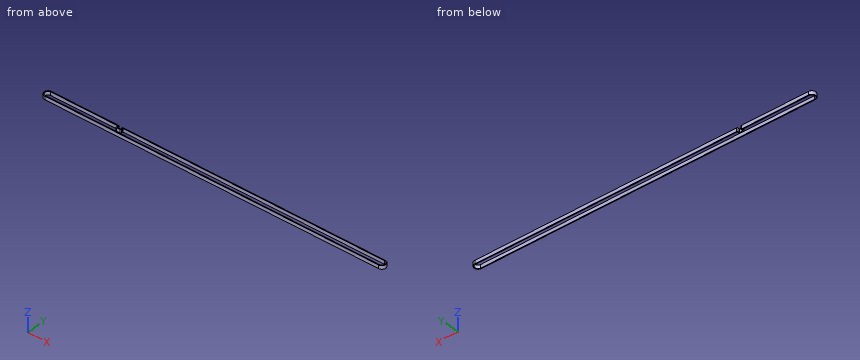
```python
from build123d import *

# Parameters (mm, degrees)
SALIENTE_EXTRUIR1_DEPTH = 6
REDONDEO1_R             = 0.3
REDONDEO2_R             = 1.2


with BuildPart() as part:
    # Croquis1 → Saliente-Extruir1 (new body)
    with BuildSketch(Plane.XY):
        with BuildLine():
            Line((0, 6.9), (120, 6.9))
            Line((120, 6.9), (120, 2.5))
            Line((120, 2.5), (126, 2.5))
            Line((126, 2.5), (126, 6.9))
            Line((126, 6.9), (590, 6.9))
            ThreePointArc((590, 6.9), (596.9, 0), (590, -6.9))
            Line((590, -6.9), (0, -6.9))
            ThreePointArc((0, -6.9), (-6.9, 0), (0, 6.9))
        make_face()
        with BuildLine():
            Line((0, 5.5), (118.6, 5.5))
            Line((118.6, 5.5), (118.6, 1.1))
            Line((118.6, 1.1), (127.4, 1.1))
            Line((127.4, 1.1), (127.4, 5.5))
            Line((127.4, 5.5), (590, 5.5))
            ThreePointArc((590, 5.5), (595.5, 0), (590, -5.5))
            Line((590, -5.5), (0, -5.5))
            ThreePointArc((0, -5.5), (-5.5, 0), (0, 5.5))
        make_face(mode=Mode.SUBTRACT)
    extrude(amount=SALIENTE_EXTRUIR1_DEPTH)

    # Redondeo1
    redondeo1_edges = [part.edges().sort_by_distance(p)[0] for p in [
        (120, 2.5, 3),
        (126, 2.5, 3),
        (127.4, 5.5, 3),
        (118.6, 5.5, 3),
    ]]
    fillet(redondeo1_edges, radius=REDONDEO1_R)

    # Redondeo2
    redondeo2_edges = [part.edges().sort_by_distance(p)[0] for p in [
        (120, 6.9, 3),
        (126, 6.9, 3),
        (127.4, 1.1, 3),
        (118.6, 1.1, 3),
    ]]
    fillet(redondeo2_edges, radius=REDONDEO2_R)


solid = part.part
```
Geometry: final body of the model. Coordinates: model frame, mm. Round coordinates to 2 decimals unless told otherwise and drop trailing zeros. Write each loop counter-clockwise with the first axis right and the second up, starting at its lowest first coordinate (ties: lowest second). Pieces come first, ordered by that corner, then holes. Notation, with made-up numbers: M 27,60 L 75,60 A25 cw 75,99 Z; hole C 86.5,75.25 d10. An arc over 180 degrees is marked long. Answer in a Markdown table with one row per item. Add a question column.
(1) Contact query for flat-ended pins moving along their axis: pin 1 (3 mm diameter, centred on y = 4, z = 3, fed in from +X); pin 2 (2.5 mm diameter, centred on y = 4, z = 4, fed in from -X); pin 3 (0.9 mm diameter, centred on y = 4, z = 3.5, fed in from -X). Output: stop coordinate, or through.
(2) Cut plane A-A, the plane x = 346.5. Return the cut outline in (y, z).
(3) Ray query, L1, parallel to Y at x = 320.5, z = 2.15; L2, parallel to X at y = 3.75, z = 3.4; L3, parallel to X at y = 1.75, z = 4.6. Return the intervals inside material, ascending.
(4) Cut plane B-B, the plane z = 2.05. Return the cut outline in (x, y), then the cut area to 3 significant figures.
Established:
| question | item | result |
|---|---|---|
| 1 | pin 1 | x = 596.43 |
| 1 | pin 2 | x = -6.33 |
| 1 | pin 3 | x = -5.92 |
| 2 | outline | M -6.9,0 L -5.5,0 L -5.5,6 L -6.9,6 Z; M 5.5,0 L 6.9,0 L 6.9,6 L 5.5,6 Z |
| 3 | L1 | -6.9 to -5.5, 5.5 to 6.9 |
| 3 | L2 | -5.79 to -4.02, 118.6 to 120, 126 to 127.4, 594.02 to 595.79 |
| 3 | L3 | -6.67 to -5.21, 118.73 to 127.27, 595.21 to 596.67 |
| 4 | outline | M 0,-6.9 L 590,-6.9 A6.9 ccw 590,6.9 L 127.2,6.9 A1.2 ccw 126,5.7 L 126,2.8 A0.3 cw 125.7,2.5 L 120.3,2.5 A0.3 cw 120,2.8 L 120,5.7 A1.2 ccw 118.8,6.9 L 0,6.9 A6.9 ccw Z; hole M 0,-5.5 L 590,-5.5 A5.5 ccw 590,5.5 L 127.7,5.5 A0.3 ccw 127.4,5.2 L 127.4,2.3 A1.2 cw 126.2,1.1 L 119.8,1.1 A1.2 cw 118.6,2.3 L 118.6,5.2 A0.3 ccw 118.3,5.5 L 0,5.5 A5.5 ccw Z |
| 4 | area | 1,720 mm² |
